Build history of the part. All positions in model axes, mm. Face numbers are marked on the shaded views. A direction names the side the tool comes from. Round coordinates to 2 decimals unless told otherwise and drop trailing zeros. Loops run counter-clockwise (first coordinate to the right, second up) from the corner with the lowest first, then second, coordinate; pieces in that order, holes last. Notation, with made-up numbers: M 68,77 L 84,77 A26 ccw 84,92 Z; hole C 87.25,15.25 d10. An arc over 180 degrees is marked long. One line per item, written item: value.
```python
from build123d import *

# Parameters (mm, degrees)
BOSS_EXTRUDE1_DEPTH      = 5
BOSS_EXTRUDE1_DEPTH_BACK = 5
CUT_EXTRUDE1_DEPTH       = 5
BOSS_EXTRUDE2_START      = -14
SKETCH3_W                = 5.881583951
SKETCH3_H                = 10
BOSS_EXTRUDE2_DEPTH      = 8
BOSS_EXTRUDE3_START      = 10
BOSS_EXTRUDE3_DEPTH      = 10
FILLET2_R                = 5
FILLET3_R                = 2
SKETCH5_R                = 2
SKETCH5_W                = 3
SKETCH5_H                = 3
CUT_EXTRUDE2_DEPTH       = 4
FILLET4_R                = 1
SKETCH6_R                = 3.25
CUT_EXTRUDE3_DEPTH       = 5
BOSS_EXTRUDE4_START      = -14
SKETCH7_R                = 2
BOSS_EXTRUDE4_DEPTH      = 3.7
FILLET5_R                = 1.6


with BuildPart() as part:
    # Sketch1 → Boss-Extrude1 (new, two sides: drawn at the far end of the back side and taken through both)
    with BuildSketch(Plane.XY.offset(-BOSS_EXTRUDE1_DEPTH_BACK)):
        Polygon((5, -10), (5, 0), (0, 0), (-5, 0), (-35, 0), (-40, 0), (-40, -14), (-31.982625312, -14), (-31.982625312, -10), (-5, -10), align=None)
        with BuildLine():
            ThreePointArc((-26.324974154, -6.579298906), (-34, -5), (-26.324974154, -3.420701094))
            Line((-26.324974154, -3.420701094), (-12.675025846, -3.420701094))
            ThreePointArc((-12.675025846, -3.420701094), (-8.193806283, -1.082085798), (-5, -5))
            ThreePointArc((-5, -5), (-8.193806283, -8.917914202), (-12.675025846, -6.579298906))
            Line((-12.675025846, -6.579298906), (-26.324974154, -6.579298906))
        make_face(mode=Mode.SUBTRACT)
    extrude(amount=BOSS_EXTRUDE1_DEPTH + BOSS_EXTRUDE1_DEPTH_BACK)

    # Sketch2 → Cut-Extrude1 (cut)
    with BuildSketch(Plane(origin=(0, 0, 0), x_dir=(1, 0, 0), z_dir=(0, 1, 0))):
        with BuildLine():
            Line((-2.520975228, 1.25), (2.520975228, 1.25))
            ThreePointArc((2.520975228, 1.25), (3.770975228, 0), (2.520975228, -1.25))
            Line((2.520975228, -1.25), (-2.520975228, -1.25))
            ThreePointArc((-2.520975228, -1.25), (-3.770975228, 0), (-2.520975228, 1.25))
        make_face()
    extrude(amount=-CUT_EXTRUDE1_DEPTH, mode=Mode.SUBTRACT)

    # Sketch3 → Boss-Extrude2 (add)
    with BuildSketch(Plane(origin=(0, 0, 0), x_dir=(1, 0, 0), z_dir=(0, 1, 0)).offset(BOSS_EXTRUDE2_START)):
        with BuildLine():
            Line((0, 20), (0, 5))
            Line((0, 5), (5.881583951, 5))
            Line((5.881583951, 5), (5.881583951, -5))
            Line((5.881583951, -5), (0, -5))
            Line((0, -5), (0, -20))
            ThreePointArc((0, -20), (14.142135624, -14.142135624), (20, 0))
            ThreePointArc((20, 0), (14.142135624, 14.142135624), (0, 20))
        make_face()
        with Locations((2.940791976, 0)):
            Rectangle(SKETCH3_W, SKETCH3_H)
        with BuildLine():
            Line((0, 5), (-19.364916731, 5))
            ThreePointArc((-19.364916731, 5), (-20, 0), (-19.364916731, -5))
            Line((-19.364916731, -5), (0, -5))
            Line((0, -5), (0, 5))
        make_face()
        with BuildLine():
            Line((-19.364916731, 5), (-40, 5))
            Line((-40, 5), (-40, -5))
            Line((-40, -5), (-19.364916731, -5))
            ThreePointArc((-19.364916731, -5), (-20, 0), (-19.364916731, 5))
        make_face()
    extrude(amount=-BOSS_EXTRUDE2_DEPTH)

    # Sketch4 → Boss-Extrude3 (add)
    with BuildSketch(Plane(origin=(0, -14, 0), x_dir=(1, 0, 0), z_dir=(0, 1, 0)).offset(BOSS_EXTRUDE3_START)):
        with BuildLine():
            ThreePointArc((20, 0), (14.142135624, 14.142135624), (0, 20))
            Line((0, 20), (0, 6))
            Line((0, 6), (6, 6))
            Line((6, 6), (6, -6))
            Line((6, -6), (0, -6))
            Line((0, -6), (0, -20))
            ThreePointArc((0, -20), (14.142135624, -14.142135624), (20, 0))
        make_face()
    extrude(amount=-BOSS_EXTRUDE3_DEPTH)

    # Fillet2
    fillet2_edges = [part.edges().sort_by_distance(p)[0] for p in [
        (-40, -11, -5),
        (-40, -11, 5),
        (6, -9, 6),
        (6, -9, -6),
        (5, -5, 5),
        (5, -5, -5),
    ]]
    fillet(fillet2_edges, radius=FILLET2_R - 0.0001)  # a hair under: the kernel refuses the full size

    # Fillet3
    fillet3_edges = [part.edges().sort_by_distance(p)[0] for p in [
        (-19.5, -3.420701094, 5),
        (-19.5, -3.420701094, -5),
        (-19.5, -6.579298906, 5),
        (-19.5, -6.579298906, -5),
        (-31.982625312, -10, 0),
        (-31.982625312, -14, 0),
        (0, -13, -20),
        (0, -13, 20),
    ]]
    fillet(fillet3_edges, radius=FILLET3_R - 0.0001)  # a hair under: the kernel refuses the full size

    # Sketch5 → Cut-Extrude2 (cut)
    with BuildSketch(Plane.XZ.offset(22)):
        with Locations(Location((0, 0, 0), (0, 0, 270))):
            Circle(SKETCH5_R)
        with BuildLine():
            Line((-35, 3.25), (-12, 3.25))
            ThreePointArc((-12, 3.25), (-8.75, 0), (-12, -3.25))
            Line((-12, -3.25), (-35, -3.25))
            ThreePointArc((-35, -3.25), (-38.25, 0), (-35, 3.25))
        make_face()
        with Locations((-5, 0)):
            Rectangle(SKETCH5_W, SKETCH5_H)
        with Locations((5, 0)):
            Rectangle(SKETCH5_W, SKETCH5_H)
    extrude(amount=-CUT_EXTRUDE2_DEPTH, mode=Mode.SUBTRACT)

    # Fillet4
    fillet4_edges = [part.edges().sort_by_distance(p)[0] for p in [
        (-23.5, -18, 3.25),
        (-8.75, -18, 0),
        (-23.5, -18, -3.25),
        (-38.25, -18, 0),
        (0, -18, -5),
        (0, -18, 5),
        (0, -22, 2),
    ]]
    fillet(fillet4_edges, radius=FILLET4_R)

    # Sketch6 → Cut-Extrude3 (cut)
    with BuildSketch(Plane.XZ.offset(22)):
        with Locations(Location((-35, 0, 0), (0, 0, 270))):
            Circle(SKETCH6_R)
    extrude(amount=-CUT_EXTRUDE3_DEPTH, mode=Mode.SUBTRACT)

    # Sketch7 → Boss-Extrude4 (add)
    with BuildSketch(Plane(origin=(0, 0, 0), x_dir=(1, 0, 0), z_dir=(0, 1, 0)).offset(BOSS_EXTRUDE4_START)):
        with Locations(Location((0, 0, 0), (0, 0, 90))):
            Circle(SKETCH7_R)
    extrude(amount=BOSS_EXTRUDE4_DEPTH)

    # Fillet5
    fillet5_edges = [part.edges().sort_by_distance(p)[0] for p in [
        (0, -14, 2),
        (0, -10.3, 2),
    ]]
    fillet(fillet5_edges, radius=FILLET5_R)


solid = part.part
```
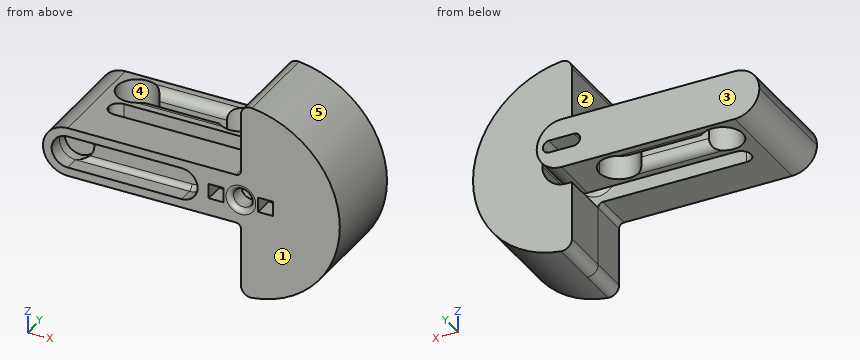
Item 1: Slice it at B-B, the plane y = -2.75. Give the number of separate pieces and of enclosed holes in the cut face, and give its area (3 significant figures).
Check values:
separate pieces: 3
enclosed holes: 1
area: 264 mm2
Item 2: Slice it at C-C, the plane z = -15.5. Give the cut face in (x, y).
Check values:
outline: M 0,-22 L 12.64,-22 L 12.64,-4 L 0,-4 Z
Item 3: Wall check: line 1 along Y through (x, z) = (-30, 1.5); line 2 along Y through (x, z) = (-19.5, -1); line 3 along X through (y, z) = (-19.35, 0). Give the ranges that are in metal, low to high.
Check values:
line 1: y = -18 to -14, -10 to -9, -1 to 0
line 2: y = -18 to -14, -10 to -6.58, -3.42 to 0
line 3: x = -40 to -38.25, -8.75 to -6.5, -3.5 to -2, 2 to 3.5, 6.5 to 20
Item 4: Which spindle directions (+Z, -Z, +X, -X, +Y, -Y) get a long thin tool onto all of the face, cutting with end or side? Do the marked faces 1 and 2. Say none if no direction does.
Check values:
face 1: +Z, -Z, +X, -X, -Y
face 2: +Z, -X, +Y, -Y
Item 5: Drop flat-ended pins along their axis: P1, Ø5, axis at x = -19.5, y = -13, coming from the +Z side; P2, Ø9.5, axis at y = -9.5, z = 10.5, coming from the -X side; P3, Ø2.5, axis at x = 5, y = -19.5, coming from the +Z side; P4, Ø8, axis at x = 0.5, y = -13, coming from the +Z side. Give the stop position or say it passes through.
Check values:
P1: stops at z = 5
P2: stops at x = 0
P3: stops at z = 19.65
P4: stops at z = 19.89
Item 6: Slice it at A-A, the plane x = -18. Give the cut face in (y, z), and give its area (3 significant figures).
Check values:
outline: M -22,-5 L -14,-5 L -14,5 L -22,5 L -22,3.25 L -19,3.25 A1 cw -18,2.25 L -18,-2.25 A1 cw -19,-3.25 L -22,-3.25 Z; M -10,-5 L -8.58,-5 A2 ccw -6.58,-3 L -6.58,3 A2 ccw -8.58,5 L -10,5 Z; M -3.42,-3 A2 ccw -1.42,-5 L 0,-5 L 0,5 L -1.42,5 A2 ccw -3.42,3 Z
area: 119 mm2
Item 7: Pull direction X, two halves, no side cores. Call the marked faces 3, 4 and 5: pulls with the +X half, pulls with the -X half, needs draft (parallel to the pull), parting line crosses it, or undercut.
Check values:
face 3: needs draft
face 4: undercut
face 5: pulls with the +X half
